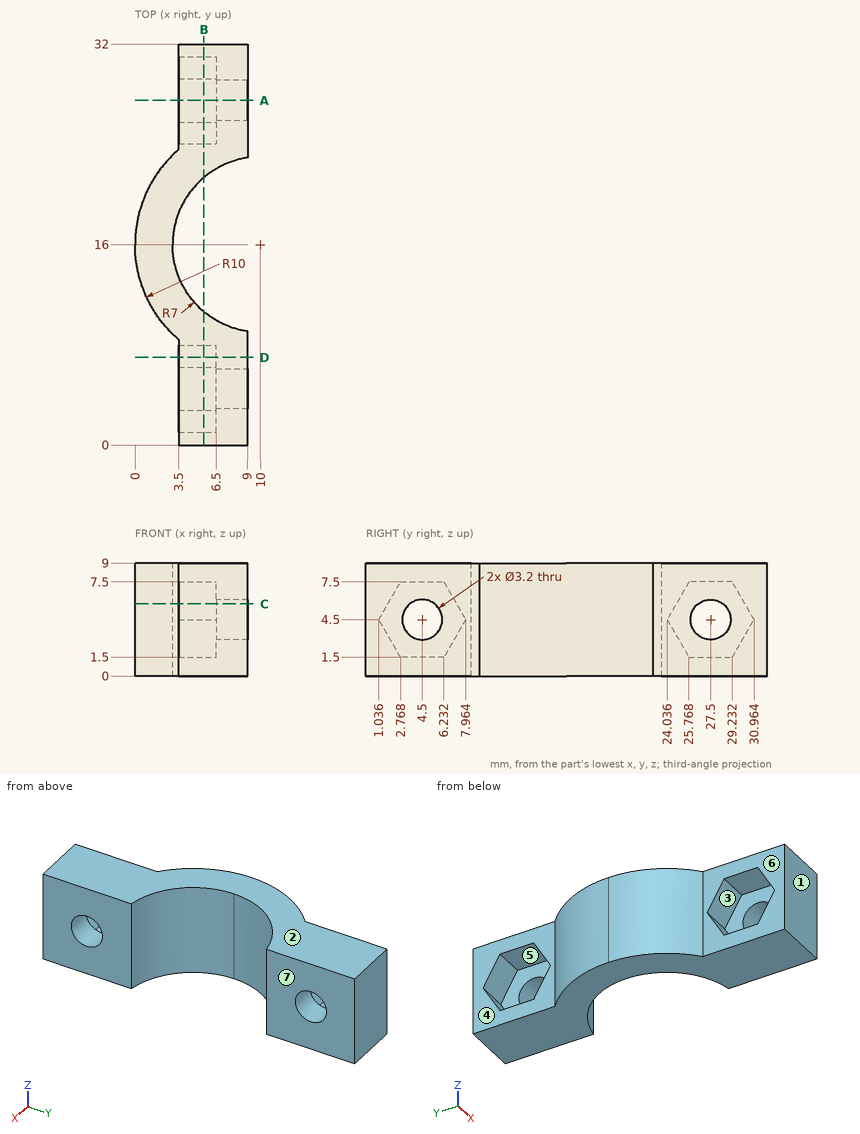
Here's the drawing with two shaded views (mm, measured from the low corner). I have some questions. A direction names the side the tool comes from. Give positions to 0.01 mm unless a question says otherwise; leave off trailing zeros. Write each loop counter-clockwise with the first axis right and the second up, starting at its lowest first coordinate (ties: lowest second). Pieces come first, ordered by that corner, then holes. Notation, with made-up numbers: (39.5, 56) -> (53.5, 56) arc R32 cw to (53.5, 93) -> close; hole circle Ø4 at (10.25, -29.5). An arc over 180 degrees is marked (long way). Use one line per item in the form item = value.
1) We'd pull the mould along Y, two halves only. Please class the marked faces 1, 2 and 3: +Y half, -Y half, draft (parallel to the pull), parting line (faces both ways), or undercut.
Verdict:
face_1 = -Y half
face_2 = draft
face_3 = undercut
2) If I drill on L1, parallel to Z at x = 7.4, y = 4.5; L2, parallel to Y at x = 4.75, z = 2.75; L3, parallel to Y at x = 6.25, z = 4.75, over which ranges is the centre line in solid material (lowest first)? Write a range as [from, to].
Verdict:
L1 = [0, 2.9], [6.1, 9]
L2 = [0, 2.05], [6.95, 11.37], [20.63, 25.05], [29.95, 32]
L3 = [0, 1.18], [7.82, 10.09], [21.91, 24.18], [30.82, 32]
3) On a 3-axis mill with a long thin cutter (end or side, diameter ignored), from which of +Z, -Z, +X, -X, +Y, -Y can I reach the whole of each face in a straight line? I mean the marked faces 4, 5, 6 and 7. Say none if no direction works.
Verdict:
face_4 = +Z, -Z, -X, +Y
face_5 = -X
face_6 = +Z, -Z, -X, -Y
face_7 = +Z, -Z, +X, +Y, -Y
4) Suppose I cut it at C-C (z = 5.75). Please give me the cut outline in (x, y), and give its area (3 significant figures).
Verdict:
outline = (3, 16) arc R7 cw to (9, 22.93) -> (9, 26.5) -> (6.5, 26.5) -> (6.5, 24.76) -> (3.5, 24.76) -> (3.5, 23.6) arc R10 ccw to (3.5, 8.4) -> (3.5, 7.24) -> (6.5, 7.24) -> (6.5, 5.5) -> (9, 5.5) -> (9, 9.07) arc R7 cw to start; (3.5, 0) -> (9, 0) -> (9, 3.5) -> (6.5, 3.5) -> (6.5, 1.76) -> (3.5, 1.76) -> close; (3.5, 30.24) -> (6.5, 30.24) -> (6.5, 28.5) -> (9, 28.5) -> (9, 32) -> (3.5, 32) -> close
area = 107 mm2
5) Suppose I cut it at B-B (x = 5.5). Please give me the cut outline in (y, z), and give its area (3 significant figures).
Verdict:
outline = (0, 0) -> (10.64, 0) -> (10.64, 9) -> (0, 9) -> close; (21.36, 0) -> (32, 0) -> (32, 9) -> (21.36, 9) -> close; hole (1.04, 4.5) -> (2.77, 1.5) -> (6.23, 1.5) -> (7.96, 4.5) -> (6.23, 7.5) -> (2.77, 7.5) -> close; hole (24.04, 4.5) -> (25.77, 1.5) -> (29.23, 1.5) -> (30.96, 4.5) -> (29.23, 7.5) -> (25.77, 7.5) -> close
area = 129 mm2
6) Suppose I cut it at D-D (y = 7). Please give me the cut outline in (x, z).
Verdict:
outline = (3.5, 0) -> (9, 0) -> (9, 9) -> (3.5, 9) -> (3.5, 6.17) -> (6.5, 6.17) -> (6.5, 2.83) -> (3.5, 2.83) -> close
7) Suppose I cut it at A-A (y = 27.5). Please give me the cut outline in (x, z), and give its area (3 significant figures).
Verdict:
outline = (3.5, 0) -> (9, 0) -> (9, 2.9) -> (6.5, 2.9) -> (6.5, 1.5) -> (3.5, 1.5) -> close; (3.5, 7.5) -> (6.5, 7.5) -> (6.5, 6.1) -> (9, 6.1) -> (9, 9) -> (3.5, 9) -> close
area = 23.5 mm2
8) I'm going to push flat-ended pins straight in: pin 1 (5 mm diameter, centred on y = 5, z = 5.5, fed in from -X); pin 2 (3.5 mm diameter, centred on y = 27.5, z = 4.5, fed in from +X); pin 3 (2 mm diameter, centred on x = 8, y = 20, fed in from +Z); pin 4 (4 mm diameter, centred on y = 4.5, z = 4.5, fed in from -X). Where does each tip first touch, or does it pass through?
Verdict:
pin_1 = 3.5
pin_2 = 9
pin_3 = through
pin_4 = 6.5
